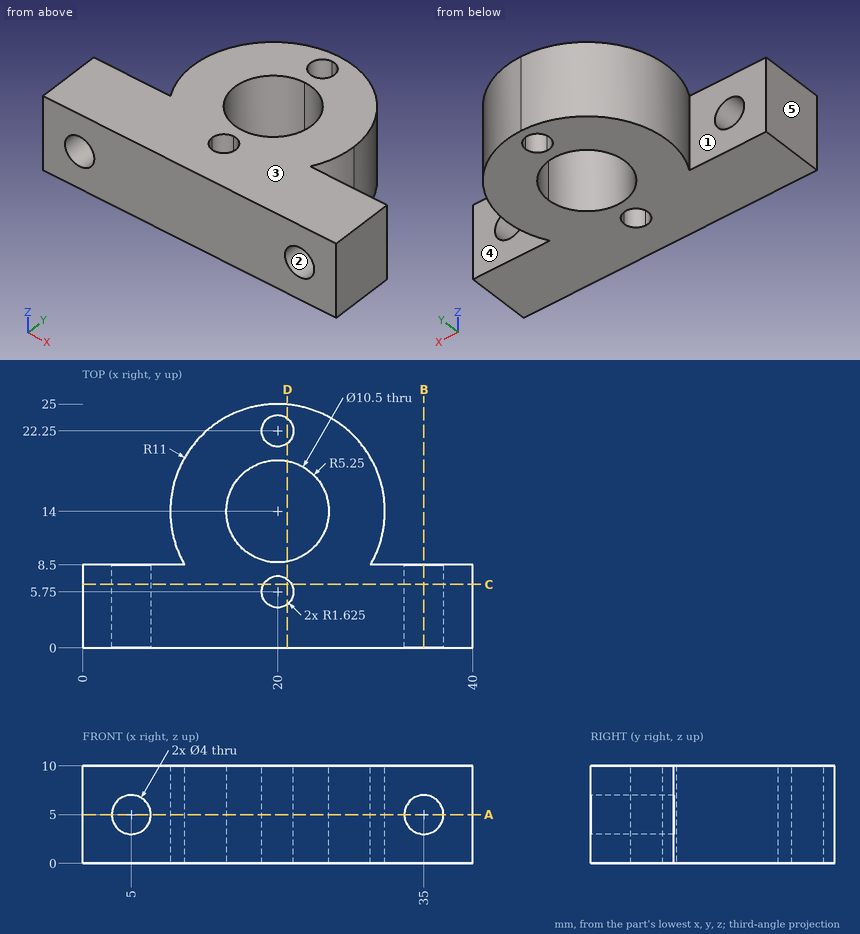
Job drawing, mm, ordinate dimensions from the low corner. One solid piece. A direction names the side the tool comes from. Coordinates: 2 decimals unless noted, no trailing zeros. Write each loop counter-clockwise with the first axis right and the second up, starting at its lowest first coordinate (ties: lowest second). Pieces come first, ordered by that corner, then holes. Notation, with made-up numbers: M 72.5,41.25 L 96.5,41.25 A25 cw 96.5,73.25 Z; hole C 48.25,56 d5. An arc over 180 degrees is marked long. Answer as a JSON object with one key per item and string values. Group by question number.
1) Wall check: line 1 (Y direction, x = 20, z = 3.75) (3 decimals); line 2 (Z direction, x = 35, y = 4); line 3 (X direction, y = 3.25, z = 6). Give the ranges that are in metal, low to high. Write a range as from..to.
2) Saw through at A-A (z = 5). Write the cut outline in (x, y) (3 decimals).
3) Saw through at C-C (y = 6.5). Write the cut outline in (x, z).
4) Mould opens along Z. For the marked faces 1, 2 and 3 say: +Z half, -Z half, draft (parallel to the pull), parting line (faces both ways), or undercut.
5) Pin check, flat tip, straight feed: pin 1 Ø3 at (x, z) = (6, 4.5) entering from +Y. Stop position of the tip, or through.
6) Tool access for the marked faces 4 and 5: list every direction of +Z, -Z, +X, -X, +Y, -Y with a clear straight run to the whole face (end or side of a thin tool).
7) Saw through at B-B (x = 35). Write the cut outline in (y, z), plus the area to 3 significant figures.
8) Saw through at D-D (x = 21). Write the cut outline in (y, z), plus the area to 3 significant figures.
Values follow:
{
 "1": {"line 1": "y = 0..4.125, 7.375..8.75, 19.25..20.625, 23.875..25", "line 2": "z = 0..3, 7..10", "line 3": "x = 0..3.27, 6.73..33.27, 36.73..40"},
 "2": {"outline": "M 0,0 L 3,0 L 3,8.5 L 0,8.5 Z; M 7,0 L 33,0 L 33,8.5 L 29.526,8.5 A11 ccw long 10.474,8.5 L 7,8.5 Z; M 37,0 L 40,0 L 40,8.5 L 37,8.5 Z; hole C 20,14 d10.5; hole C 20,5.75 d3.25; hole C 20,22.25 d3.25"},
 "3": {"outline": "M 0,0 L 18.56,0 L 18.56,10 L 0,10 Z; M 21.44,0 L 40,0 L 40,10 L 21.44,10 Z; hole C 5,5 d4; hole C 35,5 d4"},
 "4": {"face 1": "draft", "face 2": "undercut", "face 3": "+Z half"},
 "5": {"pin 1": "stops at y = 8.5"},
 "6": {"face 4": "+Z, -Z, +X", "face 5": "+Z, -Z, -X, +Y, -Y"},
 "7": {"outline": "M 0,0 L 8.5,0 L 8.5,3 L 0,3 Z; M 0,7 L 8.5,7 L 8.5,10 L 0,10 Z", "area": "51.0 mm2"},
 "8": {"outline": "M 0,0 L 4.47,0 L 4.47,10 L 0,10 Z; M 7.03,0 L 8.85,0 L 8.85,10 L 7.03,10 Z; M 19.15,0 L 20.97,0 L 20.97,10 L 19.15,10 Z; M 23.53,0 L 24.95,0 L 24.95,10 L 23.53,10 Z", "area": "95.2 mm2"}
}
